Design review of the part shown in the three views and the two pictorial views. Dimensions are in mm from the part's minimum x, y and z. Coordinates: 2 decimals unless noted, no trailing zeros. Loops run counter-clockwise (first coordinate to the right, second up) from the corner with the lowest first, then second, coordinate; pieces in that order, holes last. Notation, with made-up numbers: (-2.75, -22.5) -> (43.25, -22.5) arc R19 ccw to (43.25, -8.5) -> close; hole circle Ø2 at (33.5, 78.5). An arc over 180 degrees is marked (long way). Use CSV: the item, a comma, the result in double quotes.
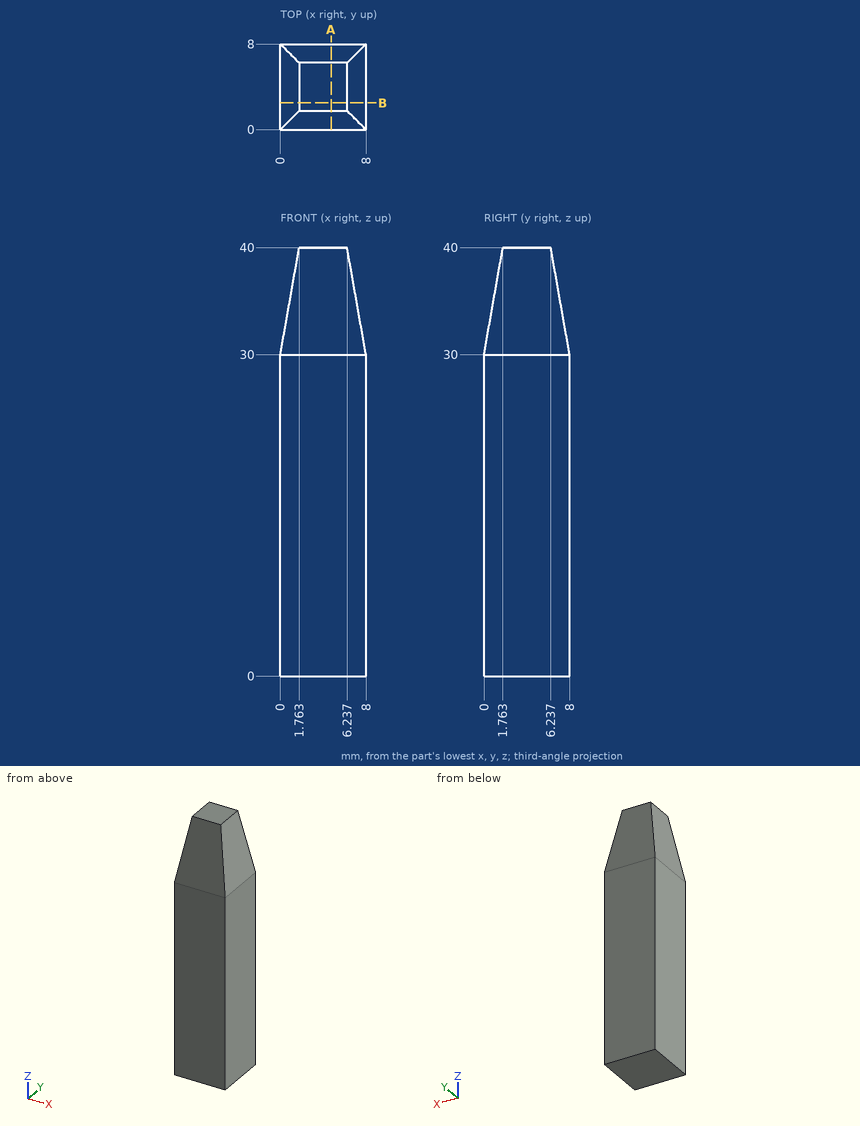
Item 1: Add section A-A (x = 4.75). Give the boundary of the cut face in (y, z), then the cut area to 3 significant figures.
Checked values:
outline,"(0, 0) -> (8, 0) -> (8, 30) -> (6.24, 40) -> (1.76, 40) -> (0, 30) -> close"
area,"302 mm^2"
Item 2: To check wall thickness, follow line 1 along Y through (x, z) = (4.75, 37) (1 decimal); line 2 along X through (y, z) = (2.5, 37.5); line 3 along Y through (x, z) = (0.5, 31). State the ranges of each line that lie inside material, in increasing order.
Checked values:
line 1,"1.2 to 6.8"
line 2,"1.32 to 6.68"
line 3,"0.18 to 7.82"
